Check sheet for the drawn part. Datum: minimum x, y, z corner. Units: mm. A direction names the side the tool comes from. Round coordinates to 2 decimals unless told otherwise and drop trailing zeros. Write each loop counter-clockwise with the first axis right and the second up, starting at its lowest first coordinate (ties: lowest second). Pieces come first, ordered by that corner, then holes. Notation, with made-up numbers: (-26, 59) -> (18, 59) arc R14 cw to (18, 69) -> close; hole circle Ø10 at (-13, 18.5). An arc over 180 degrees is marked (long way). One line per item, written item: value. Start each with the question number.
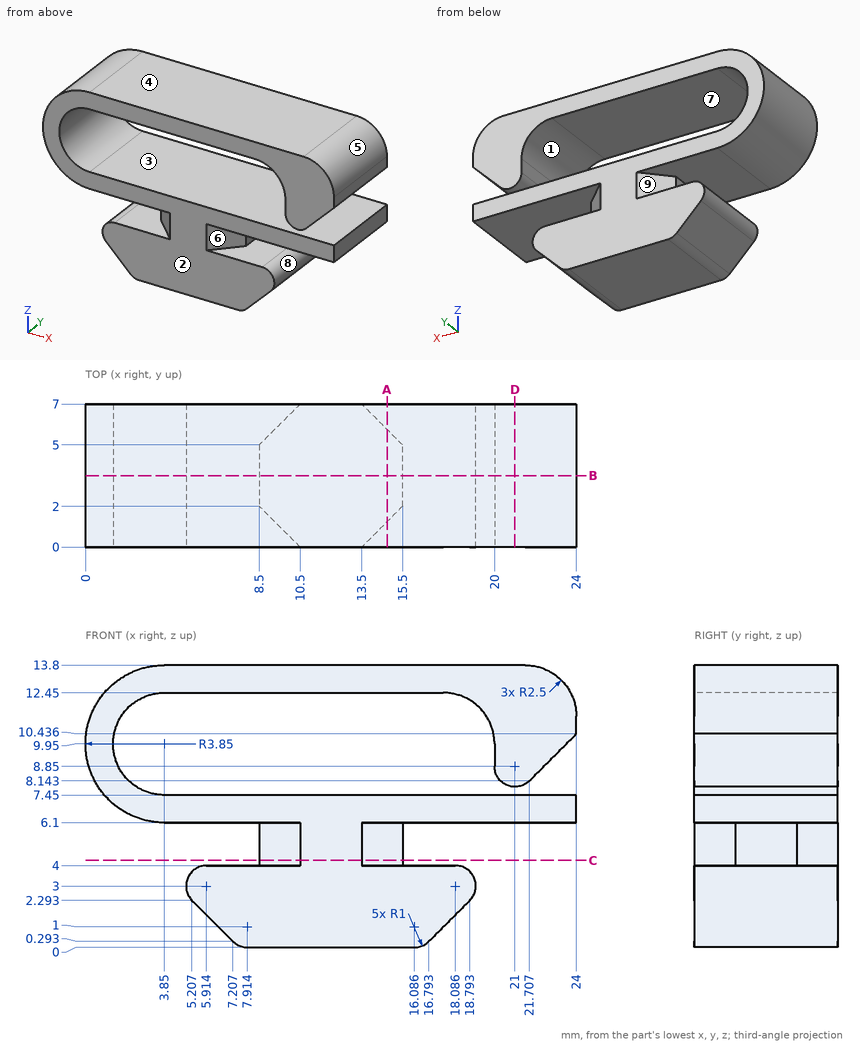
1. Cross-section at D-D (x = 21). Record the cut outline in (y, z).
2. Depth check by flat-ended pin: pin 1 Ø3 at (x, y) = (11, 3.5) entering from -Z; pin 2 Ø1.7 at (y, z) = (4, 5) entering from -X. Enter the tip coordinate at first touch or a pass-through.
3. Release check for a two-part mould opening along Z. For the marked faces 1, 2, 3 and 4 record: +Z half, -Z half, draft (parallel to the pull), parting line (faces both ways), or undercut.
4. Cross-section at A-A (x = 14.75). Record the cut outline in (y, z).
5. Cross-section at B-B (y = 3.5). Record the cut outline in (x, z).
6. Access from +Z, -Z, +X, -X, +Y, -Y to the whole of each face (thin tool, end or side, straight path). Record for the marked faces 5, 6, 7, 8 and 9.
7. Cross-section at C-C (z = 4.25). Record the cut outline in (x, y), plus the area to 3 significant figures.
8. Material ranges on probe 1 along Z at (x, y) = (8, 5.75); probe 2 along Z at (x, y) = (10.5, 1.75); probe 3 along Z at (x, y) = (6.25, 1.5), recorded low to high.
Working result:
1. outline: (0, 6.1) -> (7, 6.1) -> (7, 7.45) -> (0, 7.45) -> close; (0, 7.85) -> (7, 7.85) -> (7, 13.8) -> (0, 13.8) -> close
2. pin 1: stops at z = 0
2. pin 2: stops at x = 8.5
3. face 1: undercut
3. face 2: draft
3. face 3: undercut
3. face 4: +Z half
4. outline: (0, 0) -> (7, 0) -> (7, 4) -> (5.75, 4) -> (5.75, 6.1) -> (7, 6.1) -> (7, 7.45) -> (0, 7.45) -> (0, 6.1) -> (1.25, 6.1) -> (1.25, 4) -> (0, 4) -> close; (0, 12.45) -> (7, 12.45) -> (7, 13.8) -> (0, 13.8) -> close
5. outline: (3.85, 6.1) -> (8.5, 6.1) -> (8.5, 4) -> (5.91, 4) arc R1 ccw to (5.21, 2.29) -> (7.21, 0.29) arc R1 ccw to (7.91, 0) -> (16.09, 0) arc R1 ccw to (16.79, 0.29) -> (18.79, 2.29) arc R1 ccw to (18.09, 4) -> (15.5, 4) -> (15.5, 6.1) -> (24, 6.1) -> (24, 7.45) -> (3.85, 7.45) arc R2.5 cw to (3.85, 12.45) -> (17.5, 12.45) arc R2.5 cw to (20, 9.95) -> (20, 8.85) arc R1 ccw to (21.71, 8.14) -> (24, 10.44) -> (24, 11.3) arc R2.5 ccw to (21.5, 13.8) -> (3.85, 13.8) arc R3.85 ccw to start
6. face 5: +Z, +X, +Y, -Y
6. face 6: +X, -Y
6. face 7: +Y, -Y
6. face 8: +X, +Y, -Y
6. face 9: -X, +Y
7. outline: (8.5, 2) -> (10.5, 0) -> (13.5, 0) -> (15.5, 2) -> (15.5, 5) -> (13.5, 7) -> (10.5, 7) -> (8.5, 5) -> close
7. area: 41.0 mm^2
8. probe 1: z = 0 to 4, 6.1 to 7.45, 12.45 to 13.8
8. probe 2: z = 0 to 7.45, 12.45 to 13.8
8. probe 3: z = 1.25 to 4, 6.1 to 7.45, 12.45 to 13.8
